Can you work these out from the model? Positions are in its coordinate system, mm. Face numbers are marked on the shaded views. A direction names the side the tool comes from. Coordinates: 2 decimals unless noted, no trailing zeros. Write each loop counter-clockwise with the first axis right and the second up, starting at its lowest first coordinate (ties: lowest second). Pieces come first, ordered by that corner, then holes. Notation, with made-up numbers: M 10.25,27 L 15.25,27 A29 ccw 15.25,64 Z; hole C -1.5,70.5 d9. An arc over 180 degrees is marked long. Answer as a JSON object with one key per item and string values. Group by question number.
from build123d import *

# Parameters (mm, degrees)
PAD_DEPTH       = 58
SKETCH001_R     = 4
POCKET_DEPTH    = 25
SKETCH002_W     = 28
SKETCH002_H     = 25
POCKET001_DEPTH = 50.5
SKETCH003_R     = 5
SKETCH003_R_2   = 1.5
POCKET002_DEPTH = 58.001
POCKET003_DEPTH = 27
SKETCH005_R     = 2
SKETCH005_R_2   = 1.5
POCKET004_DEPTH = 7.501
CHAMFER_SIZE    = 2
CHAMFER001_SIZE = 3
CHAMFER002_SIZE = 3


with BuildPart() as part:
    # Sketch → Pad (new body)
    with BuildSketch(Plane.XY):
        Polygon((0, 32.5), (0, 14.5), (27, 14.5), (27, 0), (55, 0), (55, 25), (118, 25), (118, 32.5), align=None)
    extrude(amount=PAD_DEPTH)

    # Sketch001 (on Face1 of Pad) → Pocket (cut)
    with BuildSketch(Plane(origin=(0, 0, 0), x_dir=(0, -1, 0), z_dir=(-1, 0, 0))):
        with Locations((-23.5, 49)):
            Circle(SKETCH001_R)
        with Locations((-23.5, 9)):
            Circle(SKETCH001_R)
    extrude(amount=-POCKET_DEPTH, mode=Mode.SUBTRACT)

    # Sketch002 (on Face3 of Pocket) → Pocket001 (cut)
    with BuildSketch(Plane(origin=(0, 0, 0), x_dir=(1, 0, 0), z_dir=(0, 0, -1))):
        with Locations((41, -12.5)):
            Rectangle(SKETCH002_W, SKETCH002_H)
    extrude(amount=-POCKET001_DEPTH, mode=Mode.SUBTRACT)

    # Sketch003 (on Face4 of Pocket001) → Pocket002 (cut, through all)
    with BuildSketch(Plane.XY.offset(58)):
        with Locations((41, 14)):
            Circle(SKETCH003_R)
        with Locations((35.343146, 19.656854)):
            Circle(SKETCH003_R_2)
        with Locations((46.656854, 19.656854)):
            Circle(SKETCH003_R_2)
        with Locations((46.656854, 8.343146)):
            Circle(SKETCH003_R_2)
        with Locations((35.343146, 8.343146)):
            Circle(SKETCH003_R_2)
    extrude(amount=-POCKET002_DEPTH, mode=Mode.SUBTRACT)

    # Sketch004 (on Face1 of Pocket002) → Pocket003 (cut)
    with BuildSketch(Plane(origin=(0, 0, 0), x_dir=(0, -1, 0), z_dir=(-1, 0, 0))):
        Polygon((-14.5, 45.062178), (-14.5, 12.937822), (-25, 19), (-25, 39), align=None)
    extrude(amount=-POCKET003_DEPTH, mode=Mode.SUBTRACT)

    # Sketch005 (on Face13 of Pocket003) → Pocket004 (cut, through all)
    with BuildSketch(Plane.XZ.offset(-25)):
        with Locations((67, 38)):
            Circle(SKETCH005_R)
        with Locations((91, 38)):
            Circle(SKETCH005_R)
        with Locations((91, 20)):
            Circle(SKETCH005_R)
        with Locations((67, 20)):
            Circle(SKETCH005_R)
        with Locations((99.25, 29)):
            Circle(SKETCH005_R_2)
        with Locations((111.75, 29)):
            Circle(SKETCH005_R_2)
    extrude(amount=-POCKET004_DEPTH, mode=Mode.SUBTRACT)

    # Chamfer
    chamfer_edges = [part.edges().sort_by_distance(p)[0] for p in [
        (0, 23.5, 58),
        (0, 23.5, 0),
    ]]
    chamfer(chamfer_edges, length=CHAMFER_SIZE)

    # Chamfer001
    chamfer001_edges = [part.edges().sort_by_distance(p)[0] for p in [
        (27, 0, 54.25),
        (55, 0, 54.25),
    ]]
    chamfer(chamfer001_edges, length=CHAMFER001_SIZE)

    # Chamfer002
    chamfer002_edges = [part.edges().sort_by_distance(p)[0] for p in [
        (118, 28.75, 0),
        (118, 28.75, 58),
    ]]
    chamfer(chamfer002_edges, length=CHAMFER002_SIZE)


solid = part.part
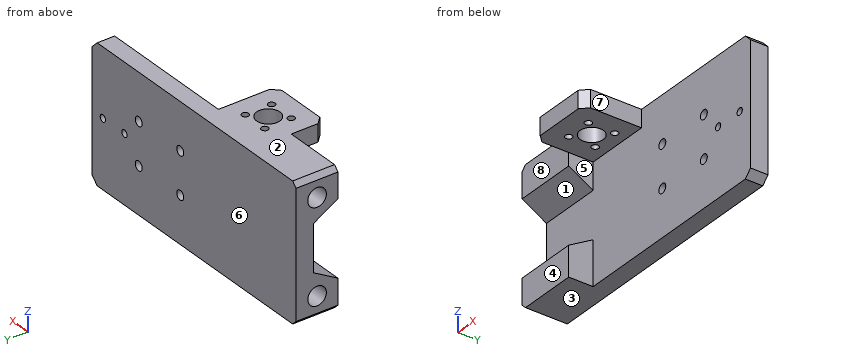
Q1. We'd pull the mould along Z, two halves only. Please class the marked faces 1, 2, 3 and 4: pulls with the +Z half, pulls with the -Z half, needs draft (parallel to the pull), parting line crosses it, or undercut.
Q2. On a 3-axis mill with a long thin cutter (end or side, diameter ignored), from which of +Z, -Z, +X, -X, +Y, -Y can I reach the whole of each face in a straight line? I mean the marked faces 5, 6, 7 and 8. Say none if no direction works.
Q3. If we section it at B-B on z = 29: List the corners of the cut face in (x, y) for me.
Q4. If we section it at C-C on x = 23.5: List the corners of the cut face in (y, z) for me, and give its area (3 significant figures).
Q5. If we section it at A-A on x = 67: List the corners of the cut face in (y, z) for me, and give its area (3 significant figures).
Q6. Please list where these lines run through material, in increasing order: L1, parallel to Z at x = 91, y = 29.75; L2, parallel to Y at x = 41, z = 54.5; L3, parallel to Z at x = 13.5, y = 23.5.
Q7. Will these pins go through, and if not, where does the flat tip stop? pin 1 (3.5 mm diameter, centred on x = 46.66, y = 8.34, fed in from -Z); pin 2 (4 mm diameter, centred on y = 25, z = 49, fed in from -X); pin 3 (1.5 mm diameter, centred on y = 25.5, z = 41.5, fed in from -X); pin 4 (11.5 mm diameter, centred on y = 17.5, z = 11.5, fed in from +X).
Q8. If we section it at D-D on y = 23.5: List the corners of the cut face in (x, z) for me, and give its area (3 significant figures).
Reply:
{
 "1": {"face 1": "undercut", "face 2": "pulls with the +Z half", "face 3": "pulls with the -Z half", "face 4": "needs draft"},
 "2": {"face 5": "-Z, +X, -Y", "face 6": "+Z, -Z, +X, -X, +Y", "face 7": "+Z, -Z, +X, -Y", "face 8": "+Z, -Z, -X, -Y"},
 "3": {"outline": "M 0,25 L 97.75,25 L 97.75,32.5 L 0,32.5 Z; M 100.75,25 L 110.25,25 L 110.25,32.5 L 100.75,32.5 Z; M 113.25,25 L 118,25 L 118,32.5 L 113.25,32.5 Z"},
 "4": {"outline": "M 14.5,0 L 32.5,0 L 32.5,58 L 14.5,58 L 14.5,45.06 L 25,39 L 25,19 L 14.5,12.94 Z; hole C 23.5,9 d8; hole C 23.5,49 d8", "area": "670 mm^2"},
 "5": {"outline": "M 25,0 L 32.5,0 L 32.5,18 L 25,18 Z; M 25,22 L 32.5,22 L 32.5,36 L 25,36 Z; M 25,40 L 32.5,40 L 32.5,58 L 25,58 Z", "area": "375 mm^2"},
 "6": {"L1": "0 to 18, 22 to 36, 40 to 58", "L2": "0 to 9, 19 to 32.5", "L3": "0 to 5, 13 to 18.13, 39.87 to 45, 53 to 58"},
 "7": {"pin 1": "z = 50.5", "pin 2": "x = 25", "pin 3": "x = 0", "pin 4": "x = 27"},
 "8": {"outline": "M 0,2 L 2,0 L 27,0 L 27,18.13 L 0,18.13 L 0,13 L 25,13 L 25,5 L 0,5 Z; M 0,39.87 L 27,39.87 L 27,50.5 L 55,50.5 L 55,58 L 2,58 L 0,56 L 0,53 L 25,53 L 25,45 L 0,45 Z", "area": "785 mm^2"}
}
